Input: part model. Units: mm. Frame: model coordinates. Coordinates: 2 decimals unless noted, no trailing zeros. Write each loop counter-clockwise with the first axis right and the second up, starting at its lowest first coordinate (ties: lowest second). Pieces come first, ordered by that corner, then holes. Notation, with made-up numbers: (42.5, 62.5) - (68.5, 62.5) arc R20 cw to (68.5, 79.5) - close; hole circle Ø3 at (72.5, -34.5). An arc over 180 degrees is marked (long way). Use CSV: the item, a comma, the result in double quotes.
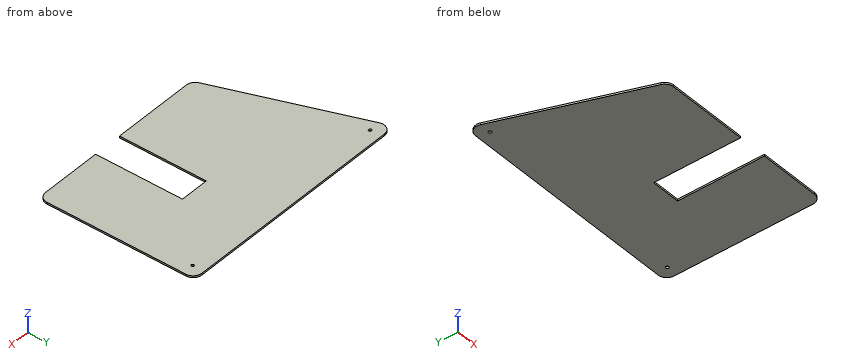
```python
from build123d import *

# Parameters (mm, degrees)
BASE_FLANGE1_DEPTH = 3.175
FILLET1_R          = 15
SKETCH2_W          = 50
SKETCH2_H          = 150
CUT_EXTRUDE1_DEPTH = 10
SKETCH3_R          = 2.5
CUT_EXTRUDE2_DEPTH = 10


# Sheet-metal steps are written as plain solids
with BuildPart() as part:
    # Sketch1 → Base-Flange1 (new body)
    with BuildSketch(Plane.XY):
        Polygon((0, 270), (0, 0), (-321.154386438, 0), (-419.42634969, 270), align=None)
    extrude(amount=-BASE_FLANGE1_DEPTH)

    # Fillet1
    fillet1_edges = [part.edges().sort_by_distance(p)[0] for p in [
        (0, 270, -1.5875),
        (0, 0, -1.5875),
        (-321.154386438, 0, -1.5875),
        (-419.42634969, 270, -1.5875),
    ]]
    fillet(fillet1_edges, radius=FILLET1_R)

    # Sketch2 → Cut-Extrude1 (cut)
    with BuildSketch(Plane(origin=(0, 0, -3.175), x_dir=(-1, 0, 0), z_dir=(0, 0, -1))):
        with Locations((145, 75)):
            Rectangle(SKETCH2_W, SKETCH2_H)
    extrude(amount=-CUT_EXTRUDE1_DEPTH, mode=Mode.SUBTRACT)

    # Sketch3 → Cut-Extrude2 (cut)
    with BuildSketch(Plane(origin=(0, 0, -3.175), x_dir=(-1, 0, 0), z_dir=(0, 0, -1))):
        with Locations((20, 250)):
            Circle(SKETCH3_R)
        with Locations((392.099518901, 250)):
            Circle(SKETCH3_R)
    extrude(amount=-CUT_EXTRUDE2_DEPTH, mode=Mode.SUBTRACT)


solid = part.part
```
(1) Cut plane A-A on z = -1.7. Return loops of the section in (x, y), and give its area (3 significant figures).
Check values:
outline,"(-412.1, 249.87) - (-324.75, 9.87) arc R15 ccw to (-310.65, 0) - (-170, 0) - (-170, 150) - (-120, 150) - (-120, 0) - (-15, 0) arc R15 ccw to (0, 15) - (0, 255) arc R15 ccw to (-15, 270) - (-398, 270) arc R15 ccw to start; hole circle Ø5 at (-392.1, 250); hole circle Ø5 at (-20, 250)"
area,"92,200 mm^2"
(2) Cut plane B-B on y = 71. Return loops of the section in (x, z) (3 decimals).
Check values:
outline,"(-346.996, -3.175) - (-170, -3.175) - (-170, 0) - (-346.996, 0) - close; (-120, -3.175) - (0, -3.175) - (0, 0) - (-120, 0) - close"
(3) Cut plane D-D on y = 214. Return loops of the section in (x, z) (3 decimals).
Check values:
outline,"(-399.044, -3.175) - (0, -3.175) - (0, 0) - (-399.044, 0) - close"
(4) Ray query, probe 1 along X at (y, z) = (250, -2); probe 2 along Y at (x, z) = (-20, -0.7); probe 3 along Y at (x, z) = (-18, -0.75). Return the intervals inside material, ascending. Write a range as from..to.
Check values:
probe 1,"-412.15..-394.6, -389.6..-22.5, -17.5..0"
probe 2,"0..247.5, 252.5..270"
probe 3,"0..248.5, 251.5..270"
(5) Cut plane C-C on x = -153. Return loops of the section in (y, z) (3 decimals), and give its area (3 significant figures).
Check values:
outline,"(150, -3.175) - (270, -3.175) - (270, 0) - (150, 0) - close"
area,"381 mm^2"
